```python
from build123d import *

# Parameters (mm, degrees)
SKETCH_1_R          = 47.5
EXTRUDE_1_DEPTH     = 63
CUT_EXTRUDE_1_DEPTH = 102.432243394
CUT_EXTRUDE_2_DEPTH = 102.432243394


with BuildPart() as part:
    # Эскиз1 → Бобышка-Вытянуть1 (new, symmetric)
    with BuildSketch(Plane(origin=(0, 0, 0), x_dir=(0, 0, -1), z_dir=(1, 0, 0))):
        Circle(SKETCH_1_R)
    extrude(amount=EXTRUDE_1_DEPTH, both=True)

    # Эскиз2 → Вырез-Вытянуть1 (cut, through all)
    with BuildSketch(Plane(origin=(-13, 0, 0), x_dir=(0, 0, -1), z_dir=(1, 0, 0))):
        with BuildLine():
            Line((-8, 31.8), (8, 31.8))
            Line((8, 31.8), (8, 26.310644234))
            ThreePointArc((8, 26.310644234), (0, -27.5), (-8, 26.310644234))
            Line((-8, 26.310644234), (-8, 31.8))
        make_face()
    extrude(amount=-CUT_EXTRUDE_1_DEPTH, mode=Mode.SUBTRACT)

    # Эскиз3 → Вырез-Вытянуть2 (cut, through all)
    with BuildSketch(Plane(origin=(13, 0, 0), x_dir=(0, 0, -1), z_dir=(1, 0, 0))):
        with BuildLine():
            Line((-7, 26.30340478), (7, 26.30340478))
            Line((7, 26.30340478), (7, 21.38340478))
            ThreePointArc((7, 21.38340478), (0, -22.5), (-7, 21.38340478))
            Line((-7, 21.38340478), (-7, 26.30340478))
        make_face()
    extrude(amount=CUT_EXTRUDE_2_DEPTH, mode=Mode.SUBTRACT)


solid = part.part
```
Part model, mm, in its own coordinate system. A direction names the side the tool comes from. Round coordinates to 2 decimals unless told otherwise and drop trailing zeros. Loops run counter-clockwise (first coordinate to the right, second up) from the corner with the lowest first, then second, coordinate; pieces in that order, holes last. Notation, with made-up numbers: (-27, 9) -> (-4, 9) arc R12 cw to (-4, 32) -> close; hole circle Ø10 at (-28.5, 35). An arc over 180 degrees is marked (long way). Use one line per item in the form item = value. Start each with the question number.
Item 1: Band-saw the part on A-A (y = 0). List the corners of the cut face in (x, z).
Item 2: Band-saw the part on B-B (x = -44). List the corners of the cut face in (y, z), plus the area to 3 significant figures.
Item 3: Tool access for faces 4 (the flat face through (13, 2, 0)), 5 (the flat face through (63, -9.9, -20.4)), 6 (the cylindrical face through (-37.65, -27.478, -1.096)): list every direction of +Z, -Z, +X, -X, +Y, -Y with a clear straight run to the whole face (end or side of a thin tool).
Item 4: Band-saw the part on D-D (x = -4.5). List the corners of the cut face in (y, z), plus the area to 3 significant figures.
Item 5: Two-plate mould, pull along Y, no slides. Class faces 1 (the flat face through (-63, -20, -20)), 2 (the cylindrical face through (0.88, -46.37, 10.3)), 3 (the flat face through (-13, 3, 0)): released by +Y, released by -Y, zero draft, split by the parting line, or undercut.
Item 6: Band-saw the part on C-C (z = 0). List the corners of the cut face in (x, y), plus the area to 3 significant figures.
Item 7: Drop flat-ended pins along their axis: pin 1 Ø8 at (x, z) = (-26.5, -1.5) entering from -Y; pin 2 Ø2.5 at (x, y) = (38.5, 24.5) entering from -Z; pin 3 Ø5 at (x, y) = (-40, 15.5) entering from -Z. Give the stop position or say it passes through.
Item 8: Drill centre lines: line 1 along Y through (x, z) = (-44, 0); line 2 along Y through (x, z) = (36, 0); line 3 along X through (y, z) = (2, 22.5). Where is each one in solid material? Low to high.
Data:
q1.outline = (-63, -47.5) -> (63, -47.5) -> (63, -22.5) -> (13, -22.5) -> (13, 22.5) -> (63, 22.5) -> (63, 47.5) -> (-63, 47.5) -> (-63, 27.5) -> (-13, 27.5) -> (-13, -27.5) -> (-63, -27.5) -> close
q2.outline = circle Ø95 at (0, 0); hole (26.31, -8) -> (31.8, -8) -> (31.8, 8) -> (26.31, 8) arc R27.5 ccw (long way) to start
q2.area = 4,640 mm^2
q3.face_4 = +X
q3.face_5 = +Z, -Z, +X, +Y, -Y
q3.face_6 = -X
q4.outline = circle Ø95 at (0, 0)
q4.area = 7,090 mm^2
q5.face_1 = zero draft
q5.face_2 = split by the parting line
q5.face_3 = undercut
q6.outline = (-63, -47.5) -> (63, -47.5) -> (63, -22.5) -> (13, -22.5) -> (13, 26.3) -> (63, 26.3) -> (63, 47.5) -> (-63, 47.5) -> (-63, 31.8) -> (-13, 31.8) -> (-13, -27.5) -> (-63, -27.5) -> close
q6.area = 6,560 mm^2
q7.pin_1 = -47.5
q7.pin_2 = -41.42
q7.pin_3 = -45.69
q8.line_1 = -47.5 to -27.5, 31.8 to 47.5
q8.line_2 = -47.5 to -22.5, 26.3 to 47.5
q8.line_3 = -13 to 63
